from build123d import *

# Parameters (mm, degrees)
SKETCH1_W                                       = 106.8
SKETCH1_H                                       = 96
SKETCH1_W_2                                     = 100.8
SKETCH1_H_2                                     = 90
BASE_DEPTH                                      = 5
BOSS_EXTRUDE1_DEPTH                             = 5
CHAMFER1_SIZE                                   = 10
FILLET1_R                                       = 10
CHAMFER4_SIZE                                   = 5
FILLET2_START                                   = -1
FILLET2_DEPTH                                   = 7
CBORE_FOR_M3_SOCKET_HEAD_CAP_SCREW1_D           = 3.9
CBORE_FOR_M3_SOCKET_HEAD_CAP_SCREW1_CBORE_D     = 6.8
CBORE_FOR_M3_SOCKET_HEAD_CAP_SCREW1_CBORE_DEPTH = 3.4
SKETCH8_W                                       = 20
SKETCH8_H                                       = 30
SKETCH8_W_2                                     = 40
SKETCH8_H_2                                     = 20
SKETCH8_W_3                                     = 26
SKETCH8_H_3                                     = 9.7
CUT_EXTRUDE1_DEPTH                              = 2.7
CUT_EXTRUDE2_START                              = 2.5
CUT_EXTRUDE2_OUTLINE_R                          = 1.55
CUT_EXTRUDE2_OUTLINE_R_2                        = 1.45
CUT_EXTRUDE2_DEPTH                              = 3.5
CUT_EXTRUDE3_START                              = -3.8
SKETCH9_3_R                                     = 1.45
CUT_EXTRUDE3_DEPTH                              = 3.8


with BuildPart() as part:
    # Sketch1 → Base (new body)
    # profile 1 of 2: a face of its own
    with BuildSketch(Plane(origin=(0, 0, 0), x_dir=(1, 0, 0), z_dir=(0, 1, 0))):
        Rectangle(SKETCH1_W, SKETCH1_H)
        Rectangle(SKETCH1_W_2, SKETCH1_H_2, mode=Mode.SUBTRACT)
    # profile 2 of 2: a face of its own
    with BuildSketch(Plane(origin=(0, 0, 0), x_dir=(1, 0, 0), z_dir=(0, 1, 0))):
        Rectangle(SKETCH1_W_2, SKETCH1_H_2)
    extrude(amount=BASE_DEPTH)

    # Sketch7 → Boss-Extrude1 (add)
    with BuildSketch(Plane.XZ):
        Polygon((53.4, -28), (71.4, -28), (71.4, -66), (33.4, -66), (33.4, -48), (53.4, -48), align=None)
        Polygon((-33.4, -48), (-53.4, -48), (-53.4, -28), (-71.4, -28), (-71.4, -66), (-33.4, -66), align=None)
        Polygon((-53.4, 36), (-58.4, 36), (-58.4, 53), (-41.4, 53), (-41.4, 48), (-53.4, 48), align=None)
        Polygon((41.4, 48), (53.4, 48), (53.4, 36), (58.4, 36), (58.4, 53), (41.4, 53), align=None)
    extrude(amount=-BOSS_EXTRUDE1_DEPTH)

    # Chamfer1
    chamfer1_edges = [part.edges().sort_by_distance(p)[0] for p in [
        (33.4, 2.5, -48),
        (53.4, 2.5, -28),
        (-53.4, 2.5, -28),
        (-33.4, 2.5, -48),
    ]]
    chamfer(chamfer1_edges, length=CHAMFER1_SIZE)

    # Fillet1
    # the kernel refuses this fillet: 10 mm, written as the material it takes off along each edge
    with BuildSketch(Plane(origin=(-71.4, -24.494897428, -28), x_dir=(1, 0, 0), z_dir=(0, 1, 0)), Plane(origin=(33.4, -24.494897428, -66), x_dir=(0, 0, 1), z_dir=(0, 1, 0))) as fillet1_piece_1:
        with BuildLine():
            CenterArc((10, 9.797958971), FILLET1_R, 180, 78.463040967)
            Line((0, 9.797958971), (-0.2, 9.797958971))
            Line((-0.2, 9.797958971), (-0.2, 0))
            Line((-0.2, 0), (0, -0.2))
            ThreePointArc((0, -0.2), (4, -0.2), (7.96, -0.195959179))
            Line((7.96, -0.195959179), (8, 0))
        make_face()
    extrude(amount=53.989794856, mode=Mode.SUBTRACT)
    with BuildSketch(Plane(origin=(-71.4, -25, -66), x_dir=(0, 0, 1), z_dir=(0, 1, 0)), Plane(origin=(71.4, -25, -66), x_dir=(-1, 0, 0), z_dir=(0, 1, 0))) as fillet1_piece_2:
        with BuildLine():
            CenterArc((FILLET1_R, FILLET1_R), FILLET1_R, 180, 90)
            Line((0, FILLET1_R), (-FILLET1_R * 0.02, FILLET1_R))
            Line((-FILLET1_R * 0.02, FILLET1_R), (-FILLET1_R * 0.02, -FILLET1_R * 0.02))
            Line((-FILLET1_R * 0.02, -FILLET1_R * 0.02), (FILLET1_R, -FILLET1_R * 0.02))
            Line((FILLET1_R, -FILLET1_R * 0.02), (FILLET1_R, 0))
        make_face()
    extrude(amount=55, mode=Mode.SUBTRACT)
    with BuildSketch(Plane(origin=(-33.4, -24.494897428, -66), x_dir=(-1, 0, 0), z_dir=(0, 1, 0)), Plane(origin=(71.4, -24.494897428, -28), x_dir=(0, 0, -1), z_dir=(0, 1, 0))) as fillet1_piece_3:
        with BuildLine():
            CenterArc((9.797958971, 10), FILLET1_R, 191.536959033, 78.463040967)
            Line((0, 8), (-0.195959179, 7.96))
            ThreePointArc((-0.195959179, 7.96), (-0.2, 4), (-0.2, 0))
            Line((-0.2, 0), (0, -0.2))
            Line((0, -0.2), (9.797958971, -0.2))
            Line((9.797958971, -0.2), (9.797958971, 0))
        make_face()
    extrude(amount=53.989794856, mode=Mode.SUBTRACT)

    # Chamfer4
    chamfer4_edges = [part.edges().sort_by_distance(p)[0] for p in [
        (41.4, 2.5, 48),
        (53.4, 2.5, 36),
        (-41.4, 2.5, 48),
        (-53.4, 2.5, 36),
    ]]
    chamfer(chamfer4_edges, length=CHAMFER4_SIZE - 0.0001)  # a hair under: the kernel refuses the full size

    # Fillet2: read off the stored shape, not the designer's step
    # Fillet2 outline → Fillet2 (cut)
    with BuildSketch(Plane(origin=(0, 0, 0), x_dir=(1, 0, 0), z_dir=(0, 1, 0)).offset(FILLET2_START)):
        with BuildLine():
            ThreePointArc((56.056854249, -33.656854249), (57.79103626, -36.25224104), (58.4, -39.313708499))
            Line((58.4, -39.313708499), (58.4, -36))
            Line((58.4, -36), (56.056854249, -33.656854249))
        make_face()
        with BuildLine():
            ThreePointArc((58.4, -45), (56.056854249, -50.656854249), (50.4, -53))
            Line((50.4, -53), (58.4, -53))
            Line((58.4, -53), (58.4, -45))
        make_face()
        with BuildLine():
            ThreePointArc((44.713708499, -53), (41.65224104, -52.39103626), (39.056854249, -50.656854249))
            Line((39.056854249, -50.656854249), (41.4, -53))
            Line((41.4, -53), (44.713708499, -53))
        make_face()
        with BuildLine():
            Line((-58.4, -36), (-58.4, -39.313708499))
            ThreePointArc((-58.4, -39.313708499), (-57.79103626, -36.25224104), (-56.056854249, -33.656854249))
            Line((-56.056854249, -33.656854249), (-58.4, -36))
        make_face()
        with BuildLine():
            ThreePointArc((-39.056854249, -50.656854249), (-41.65224104, -52.39103626), (-44.713708499, -53))
            Line((-44.713708499, -53), (-41.4, -53))
            Line((-41.4, -53), (-39.056854249, -50.656854249))
        make_face()
        with BuildLine():
            ThreePointArc((-50.4, -53), (-56.056854249, -50.656854249), (-58.4, -45))
            Line((-58.4, -45), (-58.4, -53))
            Line((-58.4, -53), (-50.4, -53))
        make_face()
    extrude(amount=FILLET2_DEPTH, mode=Mode.SUBTRACT)

    # CBORE for M3 Socket Head Cap Screw1 (through all)
    with Locations(Plane(origin=(0, 0, 0), x_dir=(-1, 0, 0), z_dir=(0, -1, 0))):
        with Locations((-48.7, 43.3), (-48.7, -43.3), (48.7, 43.3), (48.7, -43.3)):
            CounterBoreHole(CBORE_FOR_M3_SOCKET_HEAD_CAP_SCREW1_D / 2, CBORE_FOR_M3_SOCKET_HEAD_CAP_SCREW1_CBORE_D / 2, CBORE_FOR_M3_SOCKET_HEAD_CAP_SCREW1_CBORE_DEPTH)

    # Sketch8 → Cut-Extrude1 (cut)
    with BuildSketch(Plane.XZ):
        with Locations((-25, 10)):
            Rectangle(SKETCH8_W, SKETCH8_H)
        with Locations((25, 10)):
            Rectangle(SKETCH8_W, SKETCH8_H)
        with Locations((0, -28)):
            Rectangle(SKETCH8_W_2, SKETCH8_H_2)
        with Locations((-52.4, -55.15)):
            Rectangle(SKETCH8_W_3, SKETCH8_H_3)
        with Locations((52.4, -55.15)):
            Rectangle(SKETCH8_W_3, SKETCH8_H_3)
    extrude(amount=-CUT_EXTRUDE1_DEPTH, mode=Mode.SUBTRACT)

    # Cut-Extrude2: read off the stored shape, not the designer's step
    # Cut-Extrude2 outline → Cut-Extrude2 (cut)
    # profile 1 of 3: a face of its own
    with BuildSketch(Plane(origin=(0, 0, 0), x_dir=(1, 0, 0), z_dir=(0, 1, 0)).offset(CUT_EXTRUDE2_START)):
        with Locations((42.165, 32.2)):
            Circle(CUT_EXTRUDE2_OUTLINE_R)
        with Locations((42.165, 32.2)):
            Circle(CUT_EXTRUDE2_OUTLINE_R_2, mode=Mode.SUBTRACT)
    # profile 2 of 3: a face of its own
    with BuildSketch(Plane(origin=(0, 0, 0), x_dir=(1, 0, 0), z_dir=(0, 1, 0)).offset(CUT_EXTRUDE2_START)):
        with Locations((42.165, -32.2)):
            Circle(CUT_EXTRUDE2_OUTLINE_R)
        with Locations((42.165, -32.2)):
            Circle(CUT_EXTRUDE2_OUTLINE_R_2, mode=Mode.SUBTRACT)
    # profile 3 of 3: a face of its own
    with BuildSketch(Plane(origin=(0, 0, 0), x_dir=(1, 0, 0), z_dir=(0, 1, 0)).offset(CUT_EXTRUDE2_START)):
        with Locations((-42.165, -32.2)):
            Circle(CUT_EXTRUDE2_OUTLINE_R)
        with Locations((-42.165, -32.2)):
            Circle(CUT_EXTRUDE2_OUTLINE_R_2, mode=Mode.SUBTRACT)
    extrude(amount=CUT_EXTRUDE2_DEPTH, mode=Mode.SUBTRACT)

    # Sketch9<3> → Cut-Extrude3 (cut)
    with BuildSketch(Plane(origin=(0, 5, 0), x_dir=(1, 0, 0), z_dir=(0, 1, 0)).offset(CUT_EXTRUDE3_START)):
        with Locations(Location((-42.165, -32.2, 0), (0, 0, 270))):
            Circle(SKETCH9_3_R)
        with Locations(Location((42.165, -32.2, 0), (0, 0, 270))):
            Circle(SKETCH9_3_R)
        with Locations(Location((42.165, 32.2, 0), (0, 0, 270))):
            Circle(SKETCH9_3_R)
    extrude(amount=CUT_EXTRUDE3_DEPTH, mode=Mode.SUBTRACT)


solid = part.part
Model file for the job. Use its own axes, mm. A direction names the side the tool comes from. Round coordinates to 2 decimals unless told otherwise and drop trailing zeros. Loops run counter-clockwise (first coordinate to the right, second up) from the corner with the lowest first, then second, coordinate; pieces in that order, holes last. Notation, with made-up numbers: (75.25, 0) -> (110.25, 0) arc R19 ccw to (110.25, 19) -> close; hole circle Ø9 at (-25, 70.25). An arc over 180 degrees is marked (long way). Answer as CSV lines item,"result". Start each with the question number.
1) Slice it at C-C (z = 23). List the corners of the cut face in (x, y), plus the area to 3 significant figures.
2) Pin check, flat tips, straight feed: P1, Ø3.5, axis at x = 47.5, z = -42.5, coming from the -Y side; P2, Ø3, axis at x = 1.5, y = 2, coming from the -Z side; P3, Ø2, axis at y = 1, z = 3.5, coming from the +X side. Stop position of each tip, or through.
3) Probe line 1 along Z through (x, y) = (-48.7, 2.45); line 2 along X through (y, z) = (0.65, 12); line 3 along X through (y, z) = (2.75, -43.3). List the from-to ranges inside material, lowest first.
4) Slice it at D-D (z = 43.3). List the corners of the cut face in (x, y).
5) Tool access for faces 4 (the face through (57.78, 2.46, 36.23)), 5 (the face through (1, 5, -6)), 6 (the face through (-36.799, 2.465, -63.685)), 7 (the face through (-46.002, 1.676, -41.231)), 8 (the face through (42, 1.2, -32)): list every direction of +Z, -Z, +X, -X, +Y, -Y with a clear straight run to the whole face (end or side of a thin tool).
6) Slice it at B-B (z = -43.3). List the corners of the cut face in (x, y), plus the area to 3 significant figures.
7) Mould opens along Z. For faces 1 (the face through (1, 0, 8)), 2 (the face through (-53.4, 2, 7)), 3 (the face through (-41.63, 2.46, 52.38)) say: +Z half, -Z half, draft (parallel to the pull), parting line (faces both ways), or undercut.
8) Slice it at A-A (x = -48.7). List the corners of the cut face in (y, z), plus the area to 3 significant figures.
Filled in:
1,outline,"(-53.4, 0) -> (-35, 0) -> (-35, 2.7) -> (-15, 2.7) -> (-15, 0) -> (15, 0) -> (15, 2.7) -> (35, 2.7) -> (35, 0) -> (53.4, 0) -> (53.4, 5) -> (-53.4, 5) -> close"
1,area,"426 mm2"
2,P1,"stops at y = 3.4"
2,P2,"stops at z = -48"
2,P3,"stops at x = 53.4"
3,line 1,"z = -66 to -60, -50.3 to -46.7, -39.9 to 39.9, 46.7 to 53"
3,line 2,"x = -53.4 to -35, -15 to 15, 35 to 53.4"
3,line 3,"x = -71.4 to -52.1, -45.3 to 45.3, 52.1 to 71.4"
4,outline,"(-58.4, 0) -> (-52.1, 0) -> (-52.1, 3.4) -> (-50.65, 3.4) -> (-50.65, 5) -> (-58.4, 5) -> close; (-46.75, 3.4) -> (-45.3, 3.4) -> (-45.3, 0) -> (45.3, 0) -> (45.3, 3.4) -> (46.75, 3.4) -> (46.75, 5) -> (-46.75, 5) -> close; (50.65, 3.4) -> (52.1, 3.4) -> (52.1, 0) -> (58.4, 0) -> (58.4, 5) -> (50.65, 5) -> close"
5,face 4,"+X, +Y, -Y"
5,face 5,"+Z, -Z, +X, -X, +Y"
5,face 6,"-Z, +Y, -Y"
5,face 7,"-Y"
5,face 8,"+Y"
6,outline,"(-71.4, 0) -> (-52.1, 0) -> (-52.1, 3.4) -> (-50.65, 3.4) -> (-50.65, 5) -> (-71.4, 5) -> close; (-46.75, 3.4) -> (-45.3, 3.4) -> (-45.3, 0) -> (45.3, 0) -> (45.3, 3.4) -> (46.75, 3.4) -> (46.75, 5) -> (-46.75, 5) -> close; (50.65, 3.4) -> (52.1, 3.4) -> (52.1, 0) -> (71.4, 0) -> (71.4, 5) -> (50.65, 5) -> close"
6,area,"655 mm2"
7,face 1,"draft"
7,face 2,"undercut"
7,face 3,"+Z half"
8,outline,"(0, -66) -> (5, -66) -> (5, -45.25) -> (3.4, -45.25) -> (3.4, -46.7) -> (0, -46.7) -> (0, -50.3) -> (2.7, -50.3) -> (2.7, -60) -> (0, -60) -> close; (0, -39.9) -> (3.4, -39.9) -> (3.4, -41.35) -> (5, -41.35) -> (5, 41.35) -> (3.4, 41.35) -> (3.4, 39.9) -> (0, 39.9) -> close; (0, 46.7) -> (3.4, 46.7) -> (3.4, 45.25) -> (5, 45.25) -> (5, 53) -> (0, 53) -> close"
8,area,"510 mm2"
